Could you check a few things on this model? Use its own coordinates, in mm. A direction names the side the tool comes from. Coordinates: 2 decimals unless noted, no trailing zeros. Loops run counter-clockwise (first coordinate to the right, second up) from the corner with the lowest first, then second, coordinate; pieces in that order, holes last.
1) Imagine slicing it at C-C on y = 0. Please give me the cut outline in (x, z), plus the area to 3 significant figures.
2) For faces 1 (the face through (8, -15, 0)), 2 (the face through (-2, 4, -1.5)), 3 (the face through (14, 0, -6.5)), 4 (the face through (7, 15, 0)), which set-ups out of +Z, -Z, +X, -X, +Y, -Y let a thin tool reach every point of the face, with its end or its side?
3) Imagine slicing it at D-D on y = -10. Please give me the cut outline in (x, z).
4) If I drill on line 1 along Y through (x, z) = (13.1, -12.75); line 2 along Y through (x, z) = (0, 0.3); line 3 along X through (y, z) = (-12, -3.5), over which ranges is the centre line in solid material (lowest first)?
5) Imagine slicing it at A-A on z = -16.75. Please give me the cut outline in (x, y).
6) Thinking about a two-plate mould opening in Z: for faces 5 (the face through (14, 12, -13)), 6 (the face through (14, 17, -1.5)), 7 (the face through (13.48, 15.74, -12.91)), which applies, released by +Z, released by -Z, zero draft, split by the parting line, or undercut?
7) Imagine slicing it at B-B on z = -12.75. Please give me the cut outline in (x, y).
8) Will these pins go through, and if not, where does the flat tip stop? P1, Ø1.5, axis at x = 10.5, z = 0, coming from the -Y side; P2, Ø0.9, axis at x = 13.5, y = 17, coming from the +Z side; P3, Ø2.5, axis at x = 13, y = -5, coming from the -Z side.
Autodesk Inventor part; units mm, degrees
ref_plane "YZ Plane" through (0, 0, 0) normal (1, 0, 0) x (0, 1, 0)
ref_plane "XZ Plane" through (0, 0, 0) normal (0, 1, 0) x (-1, 0, 0)
ref_plane "XY Plane" through (0, 0, 0) normal (0, 0, 1) x (1, 0, 0)
sketch "草圖1" plane through (0, 0, 0) normal (0, 0, 1) x (1, 0, 0)
  circle A0 centre (0, 0) radius 2.5
  circle A1 centre (0, 0) radius 15
  dimension "d0" = 5
  dimension "d1" = 30
extrude "擠出1" add sketch "草圖1" along normal mid plane 3
sketch "草圖2" plane through (0, 0, -1.5) normal (0, 0, -1) x (-1, 0, 0)
  circle A0 centre (0, 0) radius 15
  circle A1 centre (0, 0) radius 2.5 construction
  line L0 (0, 15) -> (-15, 15)
  line L1 (-15, 15) -> (-15, -15)
  line L2 (-15, -15) -> (0, -15)
  line L3 (0, -15) -> (0, 15) construction
  circle A2 centre (0, 0) radius 15
  point P0 (0, -15)
  point P1 (-15, 0)
extrude "擠出2" add sketch "草圖2" against normal blind 3 contours A0 L1 L0 | L2 L1 A0
sketch "草圖3" plane through (0, 0, -1.5) normal (0, 0, -1) x (-1, 0, 0)
  arc A0 (0, -15) -> (0, 15) centre (0, 0) ccw
  line L0 (0, 15) -> (-15, 15)
  line L1 (-15, 15) -> (-15, -15)
  line L2 (-15, -15) -> (0, -15)
  circle A1 centre (0, 0) radius 2.5
  line L3 (-15, 15) -> (0, 15)
  line L4 (-12, 18) -> (-15, 18)
  line L5 (-15, 18) -> (-15, -18)
  line L6 (-15, -18) -> (-12, -18)
  line L7 (-12, -18) -> (-12, 18)
  point P0 (-15, 0)
  dimension "d13" = 36
  dimension "d14" = 3
extrude "擠出3" add sketch "草圖3" along normal blind 17.5 contours L7 L6 L5 L2 | L2 L1 L0 L7 | L0 L5 L4 L7
sketch "草圖5" plane through (0, 0, -19) normal (0, 0, -1) x (-1, 0, 0)
  line L0 (-12, -18) -> (-12, 18)
  line L1 (-12, 18) -> (-15, 18)
  line L2 (-15, 18) -> (-15, -18)
  line L3 (-15, -18) -> (-12, -18)
  line L4 (-15, 12) -> (-12, 12)
  line L5 (-12, 12) -> (-12, -12)
  line L6 (-12, -12) -> (-15, -12)
  line L7 (-15, -12) -> (-15, 12)
  point P0 (0, 0)
  point P1 (-15, 0)
  point P2 (-13.5, -12)
  point P3 (-13.5, 12)
  dimension "d15" = 24
extrude "擠出5" cut sketch "草圖5" against normal blind 12.5 contours L6 L2 L4 L0
sketch "草圖6" plane through (12, -18, -1.5) normal (-1, 0, 0) x (0, 0, 1)
  line L0 (-17.5, 30) -> (-5, 30) construction
  line L1 (-5, 30) -> (-5, 6) construction
  line L2 (-5, 6) -> (-17.5, 6) construction
  line L3 (-17.5, 0) -> (-17.5, 6) construction
  line L4 (0, 0) -> (-17.5, 0) construction
  line L5 (0, 0) -> (0, 3) construction
  line L6 (0, 33) -> (0, 3) construction
  line L7 (0, 33) -> (0, 36) construction
  line L8 (0, 36) -> (-17.5, 36) construction
  line L9 (-17.5, 30) -> (-17.5, 36) construction
  line L10 (-11.25, 36) -> (-11.25, 0) construction
  line L11 (0, 0) -> (-17.5, 0) construction
  circle A0 centre (-11.25, 32.5) radius 1.25
  circle A1 centre (-11.25, 3.5) radius 1.25
  line L12 (-11.25, 18) -> (-8.75, 18) construction
  point P0 (1.5, 18)
  point P1 (-11.25, 30)
  dimension "d18" = 2.5
  dimension "d19" = 29
extrude "擠出6" cut sketch "草圖6" against normal up to surface (3 mm away)
properties part number "Pad_2"
Filled in:
1. outline: (-15, -1.5) - (-2.5, -1.5) - (-2.5, 1.5) - (-15, 1.5) - close; (2.5, -1.5) - (12, -1.5) - (12, -6.5) - (15, -6.5) - (15, 1.5) - (2.5, 1.5) - close
1. area: 90.0 mm2
2. face 1: +Z, +X, -X, -Y
2. face 2: -Z, -X, +Y, -Y
2. face 3: -Z, +X, -X
2. face 4: +Z, +X, -X, +Y
3. outline: (-11.18, -1.5) - (12, -1.5) - (12, -6.5) - (15, -6.5) - (15, 1.5) - (-11.18, 1.5) - close
4. line 1: y = -18 to -15.75, -13.25 to -12, 12 to 13.25, 15.75 to 18
4. line 2: y = -15 to -2.5, 2.5 to 15
4. line 3: x = 12 to 15
5. outline: (12, -18) - (15, -18) - (15, -12) - (12, -12) - close; (12, 12) - (15, 12) - (15, 18) - (12, 18) - close
6. face 5: zero draft
6. face 6: released by +Z
6. face 7: undercut
7. outline: (12, -18) - (15, -18) - (15, -15.75) - (12, -15.75) - close; (12, -13.25) - (15, -13.25) - (15, -12) - (12, -12) - close; (12, 12) - (15, 12) - (15, 13.25) - (12, 13.25) - close; (12, 15.75) - (15, 15.75) - (15, 18) - (12, 18) - close
8. P1: stops at y = -15
8. P2: stops at z = -1.5
8. P3: stops at z = -6.5
